from build123d import *

# Parameters (mm, degrees)
F0_R     = 12.7
F1_DEPTH = 5.08
F3_DEPTH = 5.08
F5_DEPTH = 5.08
F7_DEPTH = 5.08
F8_D     = 15.24
F9_D     = 12.7


with BuildPart() as f1:
    # F0 (on Top) → F1 (new body)
    with BuildSketch(Plane.XY):
        Circle(F0_R)
    extrude(amount=F1_DEPTH)

    # F2 (on Top) → F3 (join)
    with BuildSketch(Plane.XY):
        with BuildLine():
            ThreePointArc((10.8174087007, 25.4269018523), (11.5752623309, 27.7701892875), (11.8315821556, 30.2196051925))
            ThreePointArc((11.8315821556, 30.2196051925), (-3.2728076401, 41.5895245615), (-10.0209587397, 23.9293967507))
            ThreePointArc((-10.0209587397, 23.9293967507), (0.8480645715, 18.4184559779), (10.8174087007, 25.4269018523))
        make_face()
        with BuildLine():
            ThreePointArc((10.8174087007, 25.4269018523), (0.8480645715, 18.4184559779), (-10.0209587397, 23.9293967507))
            Line((-10.0209587397, 23.9293967507), (-0.217736535, 0.5199406632))
            Line((-0.217736535, 0.5199406632), (10.8174087007, 25.4269018523))
        make_face()
    extrude(amount=F3_DEPTH)

    # F4 (on Top) → F5 (join)
    with BuildSketch(Plane.XY):
        with BuildLine():
            ThreePointArc((-12.2244191743, -27.7763577499), (-11.4774353607, -25.4519749313), (-11.2248354851, -23.0236146599))
            ThreePointArc((-11.2248354851, -23.0236146599), (-16.5763429957, -13.1421229656), (-27.7763577499, -12.2244191743))
            ThreePointArc((-27.7763577499, -12.2244191743), (-31.3666114242, -31.3666114242), (-12.2244191743, -27.7763577499))
        make_face()
        with BuildLine():
            ThreePointArc((-27.7763577499, -12.2244191743), (-16.5763429957, -13.1421229656), (-11.2248354851, -23.0236146599))
            ThreePointArc((-11.2248354851, -23.0236146599), (-11.4774353607, -25.4519749313), (-12.2244191743, -27.7763577499))
            Line((-12.2244191743, -27.7763577499), (0, 0))
            Line((0, 0), (-27.7763577499, -12.2244191743))
        make_face()
    extrude(amount=F5_DEPTH)

    # F6 (on Top) → F7 (join)
    with BuildSketch(Plane.XY):
        with BuildLine():
            ThreePointArc((16.5425266567, -29.9826324727), (28.4376217504, -35.1139976634), (36.3737546099, -24.874759838))
            ThreePointArc((36.3737546099, -24.874759838), (34.8057291344, -19.3339934072), (30.5667251163, -15.4366043497))
            ThreePointArc((30.5667251163, -15.4366043497), (18.1885027261, -17.5360015638), (16.5425266567, -29.9826324727))
        make_face()
        with BuildLine():
            ThreePointArc((16.5425266567, -29.9826324727), (18.1885027261, -17.5360015638), (30.5667251163, -15.4366043497))
            Line((30.5667251163, -15.4366043497), (0, 0))
            Line((0, 0), (16.5425266567, -29.9826324727))
        make_face()
    extrude(amount=F7_DEPTH)

    # F8 (through all)
    with Locations(Plane(origin=(0, 0, 0), x_dir=(1, 0, 0), z_dir=(0, 0, -1))):
        with Locations((0, -30.2196051925)):
            Hole(F8_D / 2)

    # F9 (through all)
    with Locations(Plane(origin=(0, 0, 0), x_dir=(1, 0, 0), z_dir=(0, 0, -1))):
        with Locations((-0.5756123574, 0.2878057712)):
            Hole(F9_D / 2)


solid = f1.part
Build history of the part. All positions in model axes, mm. A direction names the side the tool comes from. Coordinates: 2 decimals unless noted, no trailing zeros. Write each loop counter-clockwise with the first axis right and the second up, starting at its lowest first coordinate (ties: lowest second). Pieces come first, ordered by that corner, then holes. Notation, with made-up numbers: (-26.75, 7) -> (2.25, 7) arc R27 cw to (2.25, 38) -> close; hole circle Ø4 at (53, 45). An arc over 180 degrees is marked (long way). Use CSV: the item, a comma, the result in double quotes. Start each with the question number.
Q1. Cut at A-A, the plane x = -9. List the corners of the cut face in (y, z), then the cut area to 3 significant figures.
Q2. Flat gauge pins, fed straight in: pin 1 Ø1 at (x, z) = (2.5, 2.5) entering from -Y; pin 2 Ø2 at (y, z) = (-17, 4.5) entering from -X; pin 3 Ø3 at (x, z) = (-12.5, 1) entering from -Y; pin 4 Ø10 at (x, y) = (-0.58, -0.29) entering from +Z. Where does each tip first touch, or does it go through?
Q3. Cut at D-D, the plane y = -8. List the corners of the cut face in (x, z).
Q4. Drill centre lines: probe 1 along Y at (x, z) = (0, 3.7); probe 2 along X at (y, z) = (27, 4.65); probe 3 along X at (y, z) = (-23, 2.9). Where is each one in solid material? Low to high.
Q5. Cut at B-B, the plane z = 2.2. List the corners of the cut face in (x, y), then the cut area to 3 significant figures.
Q6. 3-axis set-ups, long thin cutter, end or side, ignore diameter. For faces 5 (the flat face through (-7.5, 17.91, 2.5)), 6 (the cylindrical face through (-31.59, -31.137, 2.504)), 7 (the flat face through (11.266, -20.419, 2.504)): which of +Z, -Z, +X, -X, +Y, -Y reach the whole face in a straight line?
Q7. Cut at C-C, the plane x = 0. List the corners of the cut face in (y, z).
Q8. Pull direction X, two halves, no side cores. Call faces 1 (the cylindrical face through (1.65, 37.66, 2.58)), 2 (the cylindrical face through (0.49, -12.69, 2.5)), 3 (the flat face through (-8, -5, 5.08)), 4 (the flat face through (7.75, 18.5, 2.5)): released by +X, released by -X, zero draft, split by the parting line, or undercut.
Checked values:
1,outline,"(-20.45, 0) -> (8.96, 0) -> (8.96, 5.08) -> (-20.45, 5.08) -> close; (21.49, 0) -> (37.9, 0) -> (37.9, 5.08) -> (21.49, 5.08) -> close"
1,area,"233 mm²"
2,pin 1,"stops at y = -12.54"
2,pin 2,"stops at x = -33.7"
2,pin 3,"stops at y = -30.63"
2,pin 4,"passes through"
3,outline,"(-18.18, 0) -> (15.84, 0) -> (15.84, 5.08) -> (-18.18, 5.08) -> close"
4,probe 1,"y = -12.7 to -6.61, 6.04 to 22.6, 37.84 to 42.05"
4,probe 2,"x = -11.39 to -6.91, 6.91 to 11.39"
4,probe 3,"x = -34.82 to -10.12, 12.69 to 36.21"
5,outline,"(-27.78, -12.22) arc R11.8 ccw (long way) to (-12.22, -27.78) -> (-5.12, -11.62) arc R12.7 ccw to (6.14, -11.12) -> (16.54, -29.98) arc R10.57 ccw (long way) to (30.57, -15.44) -> (11.34, -5.73) arc R12.7 ccw to (4.77, 11.77) -> (10.82, 25.43) arc R11.83 ccw (long way) to (-10.02, 23.93) -> (-4.91, 11.71) arc R12.7 ccw to (-11.62, -5.12) -> close; hole circle Ø15.24 at (0, 30.22); hole circle Ø12.7 at (-0.58, -0.29)"
5,area,"1,830 mm²"
6,face 5,"+Z, -Z, -X"
6,face 6,"+Z, -Z"
6,face 7,"+Z, -Z, -Y"
7,outline,"(-12.7, 0) -> (-6.61, 0) -> (-6.61, 5.08) -> (-12.7, 5.08) -> close; (6.04, 0) -> (22.6, 0) -> (22.6, 5.08) -> (6.04, 5.08) -> close; (37.84, 0) -> (42.05, 0) -> (42.05, 5.08) -> (37.84, 5.08) -> close"
8,face 1,"undercut"
8,face 2,"undercut"
8,face 3,"zero draft"
8,face 4,"released by +X"
